Geometry: final body of the model. Coordinates: model frame, mm. Face numbers are marked on the shaded views. Coordinates: 2 decimals unless noted, no trailing zeros. Write each loop counter-clockwise with the first axis right and the second up, starting at its lowest first coordinate (ties: lowest second). Pieces come first, ordered by that corner, then holes. Notation, with made-up numbers: (10.5, 30.25) -> (65.5, 30.25) arc R13 cw to (65.5, 37.25) -> close; hole circle Ø4 at (-2, -30.75). An arc over 180 degrees is marked (long way). Answer as a JSON object with one key per item and string values. Group by question number.
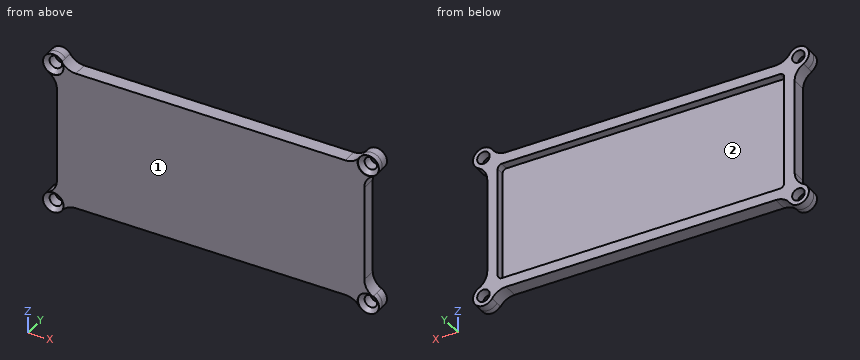
```python
from build123d import *

# Parameters (mm, degrees)
SKETCH1_R                                      = 2.5
SKETCH1_R_2                                    = 1
SKETCH1_W                                      = 73.5
SKETCH1_H                                      = 33.5
BOSS_EXTRUDE1_DEPTH                            = 1.5
SKETCH2_R                                      = 1
SKETCH2_W                                      = 68.5
SKETCH2_H                                      = 28.5
BOSS_EXTRUDE2_DEPTH                            = 2
FILLET1_R                                      = 4
CSK_FOR_M2_5_FLAT_HEAD_MACHINE_SCREW1_AT_COUNT = 2
CSK_FOR_M2_5_FLAT_HEAD_MACHINE_SCREW1_AT_PITCH = 34.329470958
CSK_FOR_M2_5_FLAT_HEAD_MACHINE_SCREW_2_COUNT   = 2
CSK_FOR_M2_5_FLAT_HEAD_MACHINE_SCREW_2_PITCH   = 75.319884043
CSK_FOR_M2_5_FLAT_HEAD_MACHINE_SCREW_3_COUNT   = 2
CSK_FOR_M2_5_FLAT_HEAD_MACHINE_SCREW_3_PITCH   = 82.774377125
FILLET2_R                                      = 1


with BuildPart() as part:
    # Sketch1 → Boss-Extrude1 (new body)
    # profile 1 of 5: a face of its own
    with BuildSketch(Plane(origin=(0, 0, 0), x_dir=(1, 0, 0), z_dir=(0, 1, 0))):
        with Locations((-37.659942021, 17.164735479)):
            Circle(SKETCH1_R)
        with Locations(Location((-37.659942021, 17.164735479, 0), (0, 0, 270))):
            Circle(SKETCH1_R_2, mode=Mode.SUBTRACT)
    # profile 2 of 5: a face of its own
    with BuildSketch(Plane(origin=(0, 0, 0), x_dir=(1, 0, 0), z_dir=(0, 1, 0))):
        with Locations((37.659942021, 17.164735479)):
            Circle(SKETCH1_R)
        with Locations(Location((37.659942021, 17.164735479, 0), (0, 0, 270))):
            Circle(SKETCH1_R_2, mode=Mode.SUBTRACT)
    # profile 3 of 5: a face of its own
    with BuildSketch(Plane(origin=(0, 0, 0), x_dir=(1, 0, 0), z_dir=(0, 1, 0))):
        with Locations((37.659942021, -17.164735479)):
            Circle(SKETCH1_R)
        with Locations(Location((37.659942021, -17.164735479, 0), (0, 0, 270))):
            Circle(SKETCH1_R_2, mode=Mode.SUBTRACT)
    # profile 4 of 5: a face of its own
    with BuildSketch(Plane(origin=(0, 0, 0), x_dir=(1, 0, 0), z_dir=(0, 1, 0))):
        with Locations((-37.659942021, -17.164735479)):
            Circle(SKETCH1_R)
        with Locations(Location((-37.659942021, -17.164735479, 0), (0, 0, 270))):
            Circle(SKETCH1_R_2, mode=Mode.SUBTRACT)
    # profile 5 of 5: a face of its own
    with BuildSketch(Plane(origin=(0, 0, 0), x_dir=(1, 0, 0), z_dir=(0, 1, 0))):
        Rectangle(SKETCH1_W, SKETCH1_H)
    extrude(amount=BOSS_EXTRUDE1_DEPTH)

    # Sketch2 → Boss-Extrude2 (add)
    with BuildSketch(Plane(origin=(0, 1.5, 0), x_dir=(1, 0, 0), z_dir=(0, 1, 0))):
        with BuildLine():
            Line((36.75, -14.836215452), (36.75, 14.836215452))
            ThreePointArc((36.75, 14.836215452), (39.599995344, 18.741502141), (35.194583126, 16.75))
            Line((35.194583126, 16.75), (-35.194583126, 16.75))
            ThreePointArc((-35.194583126, 16.75), (-39.599995344, 18.741502141), (-36.75, 14.836215452))
            Line((-36.75, 14.836215452), (-36.75, -14.836215452))
            ThreePointArc((-36.75, -14.836215452), (-39.599995344, -18.741502141), (-35.194583126, -16.75))
            Line((-35.194583126, -16.75), (35.194583126, -16.75))
            ThreePointArc((35.194583126, -16.75), (39.599995344, -18.741502141), (36.75, -14.836215452))
        make_face()
        with Locations(Location((37.659942021, -17.164735479, 0), (0, 0, 270))):
            Circle(SKETCH2_R, mode=Mode.SUBTRACT)
        with Locations(Location((37.659942021, 17.164735479, 0), (0, 0, 270))):
            Circle(SKETCH2_R, mode=Mode.SUBTRACT)
        with Locations(Location((-37.659942021, 17.164735479, 0), (0, 0, 270))):
            Circle(SKETCH2_R, mode=Mode.SUBTRACT)
        with Locations(Location((-37.659942021, -17.164735479, 0), (0, 0, 270))):
            Circle(SKETCH2_R, mode=Mode.SUBTRACT)
        Rectangle(SKETCH2_W, SKETCH2_H, mode=Mode.SUBTRACT)
    extrude(amount=BOSS_EXTRUDE2_DEPTH)

    # Fillet1
    fillet1_edges = [part.edges().sort_by_distance(p)[0] for p in [
        (36.75, 1.75, 14.836215452),
        (35.194583126, 1.75, 16.75),
        (-35.194583126, 1.75, 16.75),
        (-36.75, 1.75, 14.836215452),
        (-36.75, 1.75, -14.836215452),
        (-35.194583126, 1.75, -16.75),
        (35.194583126, 1.75, -16.75),
        (36.75, 1.75, -14.836215452),
    ]]
    fillet(fillet1_edges, radius=FILLET1_R)

    # Sketch6 → CSK for M2.5 Flat Head Machine Screw1 (revolve, cut)
    with BuildSketch(Plane(origin=(-37.659942021, 0, 17.164735479), x_dir=(0, 0, -1), z_dir=(1, 0, 0))):
        Polygon((0, 0), (0, 3.5), (1.5, 3.5), (1.5, 1.15), (2.5, 0.15), (2.5, 0), align=None)
    csk_for_m2_5_flat_head_machine_screw1 = revolve(axis=Axis((-37.659942021, -6.35, 17.164735479), (0, 1, 0)), mode=Mode.SUBTRACT)

    # CSK for M2.5 Flat Head Machine Screw1 at: CSK for M2.5 Flat Head Machine Screw1 ×2
    with Locations(*[(0, 0, -i * CSK_FOR_M2_5_FLAT_HEAD_MACHINE_SCREW1_AT_PITCH) for i in range(1, CSK_FOR_M2_5_FLAT_HEAD_MACHINE_SCREW1_AT_COUNT)]):
        add(csk_for_m2_5_flat_head_machine_screw1, mode=Mode.SUBTRACT)

    # CSK for M2.5 Flat Head Machine Screw 2: CSK for M2.5 Flat Head Machine Screw1 ×2
    with Locations(*[(i * CSK_FOR_M2_5_FLAT_HEAD_MACHINE_SCREW_2_PITCH, 0, 0) for i in range(1, CSK_FOR_M2_5_FLAT_HEAD_MACHINE_SCREW_2_COUNT)]):
        add(csk_for_m2_5_flat_head_machine_screw1, mode=Mode.SUBTRACT)

    # CSK for M2.5 Flat Head Machine Screw 3: CSK for M2.5 Flat Head Machine Screw1 ×2
    with Locations(*[Vector(0.9099420214144476, 0, -0.4147354791480819) * (i * CSK_FOR_M2_5_FLAT_HEAD_MACHINE_SCREW_3_PITCH) for i in range(1, CSK_FOR_M2_5_FLAT_HEAD_MACHINE_SCREW_3_COUNT)]):
        add(csk_for_m2_5_flat_head_machine_screw1, mode=Mode.SUBTRACT)

    # Fillet2
    fillet2_edges = [part.edges().sort_by_distance(p)[0] for p in [
        (34.25, 2.5, 14.25),
        (34.25, 2.5, -14.25),
        (-34.25, 2.5, -14.25),
        (-34.25, 2.5, 14.25),
    ]]
    fillet(fillet2_edges, radius=FILLET2_R)


solid = part.part
```
Item 1: Ray query, L1, parallel to X at y = 3.2, z = 2; L2, parallel to X at y = 0.85, z = 11.5; L3, parallel to Z at x = -9, y = 1.1. Return the intervals inside material, ascending. Write a range as [from, to].
Item 2: Section B-B on x = 18.5. Output: boundary loops of the cut face in (y, z).
Item 3: Mould query, pull axis Z, two halves, no side actions, for the marked faces 1 and 2. Classes: +Z half, -Z half, draft (parallel to the pull), parting line (faces both ways), or undercut.
Item 4: Contact query for flat-ended pins moving along their axis: pin 1 (1 mm diameter, centred on y = 1, z = 3, fed in from -X); pin 2 (2 mm diameter, centred on x = -4.5, z = -8.5, fed in from +Y); pin 3 (12 mm diameter, centred on x = -8, z = 14.5, fed in from -Y); pin 4 (2.5 mm diameter, centred on x = 37.66, z = -17.16, fed in from +Y). Output: stop coordinate, or through.
Item 5: Section A-A on z = 8. Output: boundary loops of the cut face in (x, y), then the cut area to 3 significant figures.
Answer sheet:
{
 "1": {"L1": "x = [-36.75, -34.25], [34.25, 36.75]", "L2": "x = [-36.75, 36.75]", "L3": "z = [-16.75, 16.75]"},
 "2": {"outline": "(0, -16.75) -> (3.5, -16.75) -> (3.5, -14.25) -> (1.5, -14.25) -> (1.5, 14.25) -> (3.5, 14.25) -> (3.5, 16.75) -> (0, 16.75) -> close"},
 "3": {"face 1": "draft", "face 2": "undercut"},
 "4": {"pin 1": "stops at x = -36.75", "pin 2": "stops at y = 1.5", "pin 3": "stops at y = 0", "pin 4": "passes through"},
 "5": {"outline": "(-36.75, 0) -> (36.75, 0) -> (36.75, 3.5) -> (34.25, 3.5) -> (34.25, 1.5) -> (-34.25, 1.5) -> (-34.25, 3.5) -> (-36.75, 3.5) -> close", "area": "120 mm^2"}
}
